Work out the finished part from the listing and answer in its coordinate system (mm). A direction names the side the tool comes from. Round coordinates to 2 decimals unless told otherwise and drop trailing zeros. Write each loop counter-clockwise with the first axis right and the second up, starting at its lowest first coordinate (ties: lowest second). Pieces come first, ordered by that corner, then holes.
from build123d import *

# Parameters (mm, degrees)
ESQUISSE1_W              = 46.5
ESQUISSE1_H              = 50
BOSS_EXTRU_1_DEPTH       = 5
BOSS_EXTRU_2_DEPTH       = 170
D_GAGEMENT_M41_OUTLINE_R = 2.25
D_GAGEMENT_M41_DEPTH     = 5
ENL_V_MAT_EXTRU_3_REACH  = 185.482
ESQUISSE8_W              = 4.358898944
ESQUISSE8_H              = 10.5
ENL_V_MAT_EXTRU_4_DEPTH  = 5


# Read off the part's stored shape, not the designer's step: Dégagement M41
with BuildPart() as part:
    # Esquisse1 → Boss.-Extru.1 (new body)
    with BuildSketch(Plane.XY):
        Rectangle(ESQUISSE1_W, ESQUISSE1_H)
    extrude(amount=BOSS_EXTRU_1_DEPTH)

    # Esquisse2 → Boss.-Extru.2 (add)
    with BuildSketch(Plane.XY.offset(5)):
        Polygon((-23.25, 25), (23.25, 25), (23.25, 8.5), (16.25, 8.5), (16.25, 11.5), (20.25, 11.5), (20.25, 22), (-20.25, 22), (-20.25, 11.5), (-16.25, 11.5), (-16.25, 8.5), (-23.25, 8.5), align=None)
    extrude(amount=BOSS_EXTRU_2_DEPTH)

    # Dégagement M41 outline → Dégagement M41 (cut)
    with BuildSketch(Plane.XY):
        with Locations((17.5, -18)):
            Circle(D_GAGEMENT_M41_OUTLINE_R)
        with Locations((-17.5, 0)):
            Circle(D_GAGEMENT_M41_OUTLINE_R)
        with Locations((17.5, 0)):
            Circle(D_GAGEMENT_M41_OUTLINE_R)
        with Locations((-17.5, -18)):
            Circle(D_GAGEMENT_M41_OUTLINE_R)
    extrude(amount=D_GAGEMENT_M41_DEPTH, mode=Mode.SUBTRACT)

    # Esquisse5 → Enlèv. mat.-Extru.3 (cut, up to next)
    with BuildSketch(Plane(origin=(0, 25, 0), x_dir=(1, 0, 0), z_dir=(0, 1, 0)), mode=Mode.PRIVATE) as enl_v_mat_extru_3_sk1:
        with BuildLine():
            Line((14.1, -10), (14.1, -170))
            ThreePointArc((14.1, -170), (12, -172.1), (9.9, -170))
            Line((9.9, -170), (9.9, -10))
            ThreePointArc((9.9, -10), (12, -7.9), (14.1, -10))
        make_face()
    enl_v_mat_extru_3_tool1 = extrude(enl_v_mat_extru_3_sk1.sketch, amount=-ENL_V_MAT_EXTRU_3_REACH, mode=Mode.PRIVATE) & part.part
    # Esquisse5 → Enlèv. mat.-Extru.3 (cut, up to next)
    with BuildSketch(Plane(origin=(0, 25, 0), x_dir=(1, 0, 0), z_dir=(0, 1, 0)), mode=Mode.PRIVATE) as enl_v_mat_extru_3_sk2:
        with BuildLine():
            Line((-9.9, -10), (-9.9, -170))
            ThreePointArc((-9.9, -170), (-12, -172.1), (-14.1, -170))
            Line((-14.1, -170), (-14.1, -10))
            ThreePointArc((-14.1, -10), (-12, -7.9), (-9.9, -10))
        make_face()
    enl_v_mat_extru_3_tool2 = extrude(enl_v_mat_extru_3_sk2.sketch, amount=-ENL_V_MAT_EXTRU_3_REACH, mode=Mode.PRIVATE) & part.part
    # Esquisse5 → Enlèv. mat.-Extru.3 (cut, up to next)
    with BuildSketch(Plane(origin=(0, 25, 0), x_dir=(1, 0, 0), z_dir=(0, 1, 0)), mode=Mode.PRIVATE) as enl_v_mat_extru_3_sk3:
        with BuildLine():
            Line((-5, -160), (-5, -20))
            ThreePointArc((-5, -20), (0, -15), (5, -20))
            Line((5, -20), (5, -160))
            ThreePointArc((5, -160), (0, -165), (-5, -160))
        make_face()
    enl_v_mat_extru_3_tool3 = extrude(enl_v_mat_extru_3_sk3.sketch, amount=-ENL_V_MAT_EXTRU_3_REACH, mode=Mode.PRIVATE) & part.part
    add(enl_v_mat_extru_3_tool1.solids().sort_by_distance((12, 25, 90))[0], mode=Mode.SUBTRACT)
    add(enl_v_mat_extru_3_tool2.solids().sort_by_distance((-12, 25, 90))[0], mode=Mode.SUBTRACT)
    add(enl_v_mat_extru_3_tool3.solids().sort_by_distance((0, 25, 90))[0], mode=Mode.SUBTRACT)

    # Esquisse8 → Enlèv. mat.-Extru.4 (cut)
    with BuildSketch(Plane(origin=(0, 25, 0), x_dir=(1, 0, 0), z_dir=(0, 1, 0))):
        with Locations((0, -169.75)):
            Rectangle(ESQUISSE8_W, ESQUISSE8_H)
    extrude(amount=-ENL_V_MAT_EXTRU_4_DEPTH, mode=Mode.SUBTRACT)


solid = part.part
Q1. Find section B-B (z = 117). Determine the outline of the cut face in (x, y), plus the area to 3 significant figures.
Q2. Given pin 1 (6 mm diameter, centred on x = 9, y = 19.5, fed in from +Z); pin 2 (3.5 mm diameter, centred on x = 17.5, y = -18, fed in from +Z); pin 3 (2 mm diameter, centred on x = -20.5, z = 97, fed in from -Y); pin 4 (10 mm diameter, centred on x = -5, y = -5.5, fed in from +Z), each flat-ended and moving along its own axis, determine where each tip first touches the part or whether it passes through.
Q3. Find section D-D (y = 19.5). Determine the outline of the cut face in (x, z), plus the area to 3 significant figures.
Q4. Find the intervals of material crossed by L1, parallel to Y at x = 17.5, z = 3.75; L2, parallel to X at y = 16.5, z = 57; L3, parallel to Y at x = -17, z = 14.5, in increasing order.
Q5. The mould has two halves that part along Z. Classify faces 1 (the face through (18.538, -19.996, 2.465)), 2 (the face through (5, 24, 89)), 3 (the face through (0, 0, 0)), 4 (the face through (-9.9, 24, 89)): +Z half, -Z half, draft (parallel to the pull), parting line (faces both ways), or undercut.
Q6. A tool of negligible diameter and unlimited length cuts with its end or side. For faces 5 (the face through (16.25, 10, 89)), 6 (the face through (12, 23.5, 7.9)), 7 (the face through (-18, 11.5, 89)), 8 (the face through (0, -25, 2)), 9 (the face through (20, 8.5, 89)), from which of +Z, -Z, +X, -X, +Y, -Y can it reach the whole face along a straight path? Write none if from no direction.
Q7. Find section C-C (x = -11.5). Determine the outline of the cut face in (y, z).
Q8. Find section A-A (y = -18). Determine the outline of the cut face in (x, z), plus the area to 4 significant figures.
Report:
1. outline: (-23.25, 8.5) - (-16.25, 8.5) - (-16.25, 11.5) - (-20.25, 11.5) - (-20.25, 22) - (-14.1, 22) - (-14.1, 25) - (-23.25, 25) - close; (-9.9, 22) - (-5, 22) - (-5, 25) - (-9.9, 25) - close; (5, 22) - (9.9, 22) - (9.9, 25) - (5, 25) - close; (14.1, 22) - (20.25, 22) - (20.25, 11.5) - (16.25, 11.5) - (16.25, 8.5) - (23.25, 8.5) - (23.25, 25) - (14.1, 25) - close
1. area: 189 mm2
2. pin 1: stops at z = 175
2. pin 2: passes through
2. pin 3: stops at y = 8.5
2. pin 4: stops at z = 5
3. outline: (-23.25, 0) - (23.25, 0) - (23.25, 175) - (20.25, 175) - (20.25, 5) - (-20.25, 5) - (-20.25, 175) - (-23.25, 175) - close
3. area: 1,250 mm2
4. L1: y = -25 to -20.25, -15.75 to -2.25, 2.25 to 25
4. L2: x = -23.25 to -20.25, 20.25 to 23.25
4. L3: y = 8.5 to 11.5, 22 to 25
5. face 1: draft
5. face 2: undercut
5. face 3: -Z half
5. face 4: undercut
6. face 5: +Z, -Y
6. face 6: +Y, -Y
6. face 7: +Z
6. face 8: +Z, -Z, +X, -X, -Y
6. face 9: +Z, +X, -X, -Y
7. outline: (-25, 0) - (25, 0) - (25, 7.96) - (22, 7.96) - (22, 5) - (-25, 5) - close; (22, 172.04) - (25, 172.04) - (25, 175) - (22, 175) - close
8. outline: (-23.25, 0) - (-19.75, 0) - (-19.75, 5) - (-23.25, 5) - close; (-15.25, 0) - (15.25, 0) - (15.25, 5) - (-15.25, 5) - close; (19.75, 0) - (23.25, 0) - (23.25, 5) - (19.75, 5) - close
8. area: 187.5 mm2
